```python
from build123d import *

# Parameters (mm, degrees)
SKETCH1_R           = 1.75
SKETCH1_W           = 5
SKETCH1_H           = 4
BOSS_EXTRUDE1_DEPTH = 1.6
SKETCH1_3_W         = 14
SKETCH1_3_H         = 7.5
SKETCH1_3_W_2       = 5
SKETCH1_3_H_2       = 4
BOSS_EXTRUDE2_DEPTH = 7.2
SKETCH1_5_W         = 5
SKETCH1_5_H         = 4
BOSS_EXTRUDE3_DEPTH = 1.7


with BuildPart() as part:
    # Sketch1 → Boss-Extrude1 (new body)
    with BuildSketch(Plane.XY):
        with BuildLine():
            Line((-9.722718241, 5.480077554), (-14.142135624, 9.899494937))
            ThreePointArc((-14.142135624, 9.899494937), (-14.142135624, 14.142135624), (-9.899494937, 14.142135624))
            Line((-9.899494937, 14.142135624), (-5.480077554, 9.722718241))
            ThreePointArc((-5.480077554, 9.722718241), (0, 7.452795796), (5.480077554, 9.722718241))
            Line((5.480077554, 9.722718241), (9.899494937, 14.142135624))
            ThreePointArc((9.899494937, 14.142135624), (14.142135624, 14.142135624), (14.142135624, 9.899494937))
            Line((14.142135624, 9.899494937), (9.722718241, 5.480077554))
            ThreePointArc((9.722718241, 5.480077554), (7.452795796, 0), (9.722718241, -5.480077554))
            Line((9.722718241, -5.480077554), (14.142135624, -9.899494937))
            ThreePointArc((14.142135624, -9.899494937), (14.142135624, -14.142135624), (9.899494937, -14.142135624))
            Line((9.899494937, -14.142135624), (5.480077554, -9.722718241))
            ThreePointArc((5.480077554, -9.722718241), (0, -7.452795796), (-5.480077554, -9.722718241))
            Line((-5.480077554, -9.722718241), (-9.899494937, -14.142135624))
            ThreePointArc((-9.899494937, -14.142135624), (-14.142135624, -14.142135624), (-14.142135624, -9.899494937))
            Line((-14.142135624, -9.899494937), (-9.722718241, -5.480077554))
            ThreePointArc((-9.722718241, -5.480077554), (-7.452795796, 0), (-9.722718241, 5.480077554))
        make_face()
        with Locations((-12.02081528, 12.02081528)):
            Circle(SKETCH1_R, mode=Mode.SUBTRACT)
        with Locations((12.02081528, 12.02081528)):
            Circle(SKETCH1_R, mode=Mode.SUBTRACT)
        with Locations((-12.02081528, -12.02081528)):
            Circle(SKETCH1_R, mode=Mode.SUBTRACT)
        with Locations((12.02081528, -12.02081528)):
            Circle(SKETCH1_R, mode=Mode.SUBTRACT)
        Rectangle(SKETCH1_W, SKETCH1_H, mode=Mode.SUBTRACT)
    extrude(amount=BOSS_EXTRUDE1_DEPTH)

    # Sketch1_3 → Boss-Extrude2 (add)
    with BuildSketch(Plane.XY):
        Rectangle(SKETCH1_3_W, SKETCH1_3_H)
        Rectangle(SKETCH1_3_W_2, SKETCH1_3_H_2)
    extrude(amount=BOSS_EXTRUDE2_DEPTH)

    # Sketch1_5 → Boss-Extrude3 (add)
    with BuildSketch(Plane.XY):
        Rectangle(SKETCH1_5_W, SKETCH1_5_H)
    extrude(amount=-BOSS_EXTRUDE3_DEPTH)


solid = part.part
```
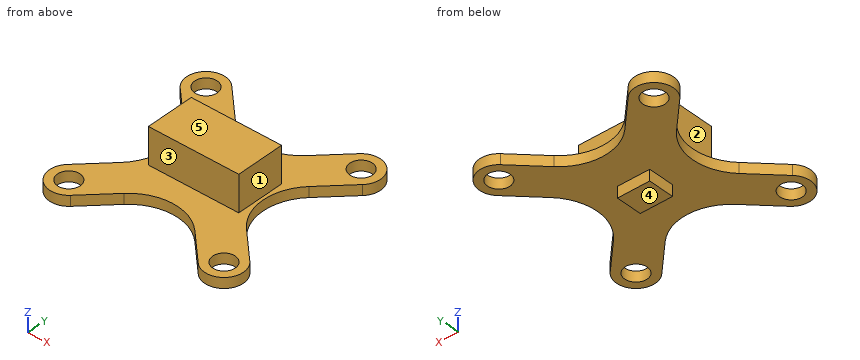
The model under review builds one solid part; all positions refer to its coordinate system, in mm. Face numbers are marked on the shaded views. A direction names the side the tool comes from. Round coordinates to 2 decimals unless told otherwise and drop trailing zeros. Order: outer loops, then holes, each group sorted by start corner. A loop starts at its lowest first (then second) coordinate and runs counter-clockwise, first axis right, second up.
(1) Tool access review of the marked faces 1, 2, 3, 4 and 5: name each direction out of +Z, -Z, +X, -X, +Y, -Y from which nothing blocks a thin tool from reaching the whole face with its end or side.
Working result:
face 1: +Z, +X, +Y, -Y
face 2: +Z, -X, +Y, -Y
face 3: +Z, +X, -X, -Y
face 4: -Z, +X, -X, +Y, -Y
face 5: +Z, +X, -X, +Y, -Y
(2) Take a section at A-A, the plane x = -8. State the section outline as (y, z) points, plus the area to 3 significant figures.
Working result:
outline: (-12.24, 0) - (-2.86, 0) - (-2.86, 1.6) - (-12.24, 1.6) - close; (2.86, 0) - (12.24, 0) - (12.24, 1.6) - (2.86, 1.6) - close
area: 30.0 mm2
(3) Wall thickness on L1, parallel to Y at x = 13, z = 1; L2, parallel to Z at x = -3.5, y = 4.5; L3, parallel to X at y = 12, z = 0.5: over which ranges is each line inside the solid? List them lowest first.
Working result:
L1: y = -14.86 to -13.47, -10.57 to -8.76, 8.76 to 10.57, 13.47 to 14.86
L2: z = 0 to 1.6
L3: x = -15.02 to -13.77, -10.27 to -7.76, 7.76 to 10.27, 13.77 to 15.02
(4) For P1, Ø3, axis at x = 1, z = 5.5, coming from the -Y side; P2, Ø1.4, axis at y = -0.5, z = -0.5, coming from the +X side; P3, Ø2, axis at x = -12.02, y = 12.02, coming from the +Z side; P4, Ø3, axis at y = -1.5, z = 5, coming from the +X side, all flat-tipped, find the tip position at first contact; note any pin that passes through.
Working result:
P1: stops at y = -3.75
P2: stops at x = 7.52
P3: passes through
P4: stops at x = 7
(5) Take a section at D-D, the plane y = 1. State the section outline as (x, z) points, plus the area to 3 significant figures.
Working result:
outline: (-7.52, 0) - (-2.5, 0) - (-2.5, -1.7) - (2.5, -1.7) - (2.5, 0) - (7.52, 0) - (7.52, 1.6) - (7, 1.6) - (7, 7.2) - (-7, 7.2) - (-7, 1.6) - (-7.52, 1.6) - close
area: 111 mm2
(6) Take a section at B-B, the plane z = 0.75. State the section outline as (x, y) points.
Working result:
outline: (-14.14, -9.9) arc R3 ccw to (-9.9, -14.14) - (-5.48, -9.72) arc R7.75 cw to (5.48, -9.72) - (9.9, -14.14) arc R3 ccw to (14.14, -9.9) - (9.72, -5.48) arc R7.75 cw to (9.72, 5.48) - (14.14, 9.9) arc R3 ccw to (9.9, 14.14) - (5.48, 9.72) arc R7.75 cw to (-5.48, 9.72) - (-9.9, 14.14) arc R3 ccw to (-14.14, 9.9) - (-9.72, 5.48) arc R7.75 cw to (-9.72, -5.48) - close; hole circle Ø3.5 at (-12.02, -12.02); hole circle Ø3.5 at (-12.02, 12.02); hole circle Ø3.5 at (12.02, -12.02); hole circle Ø3.5 at (12.02, 12.02)
(7) Take a section at C-C, the plane y = 9. State the section outline as (x, z) points.
Working result:
outline: (-13.24, 0) - (-4.65, 0) - (-4.65, 1.6) - (-13.24, 1.6) - close; (4.65, 0) - (13.24, 0) - (13.24, 1.6) - (4.65, 1.6) - close
